```python
from build123d import *

# Parameters (mm, degrees)
SKETCH1_R               = 3.175
BOSS_EXTRUDE1_DEPTH     = 1.5875
SKETCH3_W               = 50.8
SKETCH3_H               = 12.7
SKETCH3_R               = 3.175
BOSS_EXTRUDE2_DEPTH     = 1.5875
CUT_EXTRUDE1_DEPTH      = 44.12627172
CUT_EXTRUDE1_DEPTH_BACK = 44.12627172
SKETCH5_W               = 1.5875
SKETCH5_H               = 4.7625
FILLET2_R               = 0.79375
FILLET3_R               = 12.7


with BuildPart() as part:
    # Sketch1 → Boss-Extrude1 (new body)
    with BuildSketch(Plane.XY):
        with BuildLine():
            Line((-25.4, -12.7), (-12.7, -12.7))
            Line((-12.7, -12.7), (-12.7, 12.7))
            Line((-12.7, 12.7), (12.7, 12.7))
            Line((12.7, 12.7), (12.7, -12.7))
            Line((12.7, -12.7), (25.4, -12.7))
            ThreePointArc((25.4, -12.7), (38.1, 0), (25.4, 12.7))
            Line((25.4, 12.7), (25.4, 14.2875))
            Line((25.4, 14.2875), (-25.4, 14.2875))
            Line((-25.4, 14.2875), (-25.4, 12.7))
            ThreePointArc((-25.4, 12.7), (-38.1, 0), (-25.4, -12.7))
        make_face()
        with Locations((-25.4, 0)):
            Circle(SKETCH1_R, mode=Mode.SUBTRACT)
        with Locations((25.4, 0)):
            Circle(SKETCH1_R, mode=Mode.SUBTRACT)
    extrude(amount=BOSS_EXTRUDE1_DEPTH)

    # Sketch3 → Boss-Extrude2 (add)
    with BuildSketch(Plane(origin=(0, 14.2875, 0), x_dir=(1, 0, 0), z_dir=(0, 1, 0))):
        with Locations((0, 6.35)):
            Rectangle(SKETCH3_W, SKETCH3_H)
        with Locations(Location((0, 6.35, 0), (0, 0, 270))):
            Circle(SKETCH3_R, mode=Mode.SUBTRACT)
    extrude(amount=-BOSS_EXTRUDE2_DEPTH)

    # Sketch5 → Cut-Extrude1 (cut, two sides: drawn at the far end of the back side and taken through both)
    with BuildSketch(Plane.XY.offset(1.5875).offset(-CUT_EXTRUDE1_DEPTH_BACK)):
        with Locations((-24.60625, 11.90625)):
            Rectangle(SKETCH5_W, SKETCH5_H)
        with Locations((24.60625, 11.90625)):
            Rectangle(SKETCH5_W, SKETCH5_H)
    extrude(amount=CUT_EXTRUDE1_DEPTH + CUT_EXTRUDE1_DEPTH_BACK, mode=Mode.SUBTRACT)

    # Fillet2
    fillet2_edges = [part.edges().sort_by_distance(p)[0] for p in [
        (-12.7, -12.7, 0.79375),
        (-25.4, 12.7, 0.79375),
        (25.4, 12.7, 0.79375),
        (12.7, -12.7, 0.79375),
        (18.25625, 12.7, 0),
        (-18.25625, 12.7, 0),
    ]]
    fillet(fillet2_edges, radius=FILLET2_R)

    # Fillet3
    fillet3_edges = [part.edges().sort_by_distance(p)[0] for p in [
        (23.8125, 13.49375, -12.7),
        (-23.8125, 13.49375, -12.7),
    ]]
    fillet(fillet3_edges, radius=FILLET3_R - 0.0001)  # a hair under: the kernel refuses the full size


solid = part.part
```
The model under review builds one solid part; all positions refer to its coordinate system, in mm. A direction names the side the tool comes from. Round coordinates to 2 decimals unless told otherwise and drop trailing zeros. Loops run counter-clockwise (first coordinate to the right, second up) from the corner with the lowest first, then second, coordinate; pieces in that order, holes last. Notation, with made-up numbers: M 48,78.25 L 67,78.25 A12 ccw 67,97.25 Z; hole C 51.5,82 d10. An arc over 180 degrees is marked long. Put each result on its own line as item: value.
Q1. Consider section B-B, the plane x = 0. Give the boundary of the cut face in (y, z) (1 decimal), then the cut area to 3 significant figures.
Result set:
outline: M 12.7,-12.7 L 14.3,-12.7 L 14.3,-9.5 L 12.7,-9.5 Z; M 12.7,-3.2 L 14.3,-3.2 L 14.3,1.6 L 12.7,1.6 Z
area: 12.6 mm²
Q2. To check wall thickness, follow L1, parallel to Z at x = -30, y = 9.25; L2, parallel to Y at x = -4.5, z = -12; L3, parallel to X at y = 13.25, z = -6.35 (3 decimals). State the ranges of each line that lie inside material, in increasing order.
Result set:
L1: z = 0 to 1.59
L2: y = 12.7 to 14.29
L3: x = -22.111 to -3.175, 3.175 to 22.111
Q3. Consider section D-D, the plane x = 16.5. Give the boundary of the cut face in (y, z), then the cut area to 3 significant figures.
Result set:
outline: M -12.7,0 L 11.91,0 A0.79 cw 12.7,-0.79 L 12.7,-11.5 L 14.29,-11.5 L 14.29,1.59 L -12.7,1.59 Z
area: 61.2 mm²
Q4. Consider section A-A, the plane y = 0. Give the boundary of the cut face in (x, z) (1 decimal).
Result set:
outline: M -38.1,0 L -28.6,0 L -28.6,1.6 L -38.1,1.6 Z; M -22.2,0 L -12.7,0 L -12.7,1.6 L -22.2,1.6 Z; M 12.7,0 L 22.2,0 L 22.2,1.6 L 12.7,1.6 Z; M 28.6,0 L 38.1,0 L 38.1,1.6 L 28.6,1.6 Z
Q5. For pin 1 (1.7 mm diameter, centred on y = 10.5, z = 0.5, fed in from -X); pin 2 (7.5 mm diameter, centred on x = 25.4, y = 0, fed in from -Z); pin 3 (1.3 mm diameter, centred on y = 11, z = 0.5, fed in from -X); pin 4 (1.5 mm diameter, centred on x = -15.5, z = -0.5, fed in from -Y), all flat-tipped, find the tip position at first contact; note any pin that passes through.
Result set:
pin 1: stops at x = -33.66
pin 2: stops at z = 0
pin 3: stops at x = -32.76
pin 4: stops at y = -12.7
Q6. Consider section C-C, the plane z = -6.35. Give the boundary of the cut face in (x, y) (1 decimal), then the cut area to 3 significant figures.
Result set:
outline: M -22.1,12.7 L -3.2,12.7 L -3.2,14.3 L -22.1,14.3 Z; M 3.2,12.7 L 22.1,12.7 L 22.1,14.3 L 3.2,14.3 Z
area: 60.1 mm²
Q7. Machinability: for faces 5 (the flat face through (19, -12.7, 1)), 6 (the flat face through (25, 9.525, 1)), 7 (the flat face through (12.7, 1, 1)), which of the approach directions +Z, -Z, +X, -X, +Y, -Y give a long, thin tool a straight path to every point of the face, cutting with its end or side? Answer none if there is none.
Result set:
face 5: +Z, -Z, +X, -X, -Y
face 6: +Z, -Z, +Y
face 7: +Z, -Z, -Y
Q8. Mouldability with a two-part tool opening along Y and no side actions: class faces 1 (the cylindrical face through (-38.1, -0.2, 0.8)), 2 (the cylindrical face through (-22.37, 0.95, 0.78)), 3 (the cylindrical face through (28.43, 0.95, 0.78)), 4 (the flat face through (0, 14, -12.7)) as released by +Y, released by -Y, zero draft, split by the parting line, or undercut.
Result set:
face 1: split by the parting line
face 2: undercut
face 3: undercut
face 4: zero draft
